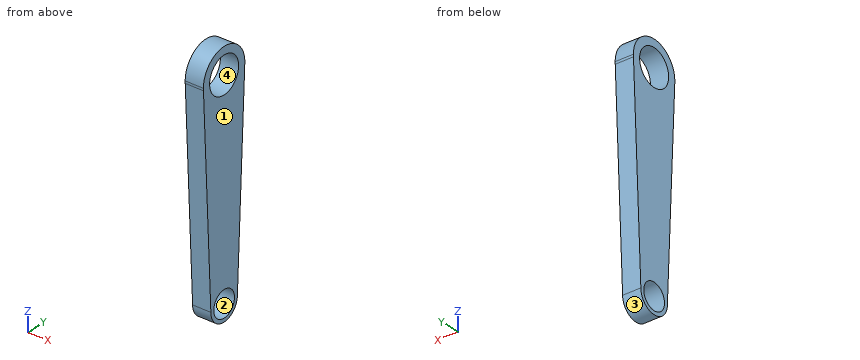
```python
from build123d import *

# Parameters (mm, degrees)
SKETCH_3_R      = 3.5
SKETCH_3_R_2    = 2.5
EXTRUDE_2_DEPTH = 3.5


with BuildPart() as part:
    # 草图3 → 凸台-拉伸2 (new body)
    with BuildSketch(Plane(origin=(0, 0, 0), x_dir=(0, 0, -1), z_dir=(1, 0, 0))):
        with BuildLine():
            Line((0.449090592, 4.979790923), (0, 5))
            ThreePointArc((0, 5), (-5, 0), (0, -5))
            Line((0, -5), (0.449090592, -4.979790923))
            Line((0.449090592, -4.979790923), (40, -3.2))
            ThreePointArc((40, -3.2), (43.2, 0), (40, 3.2))
            Line((40, 3.2), (0.449090592, 4.979790923))
        make_face()
        Circle(SKETCH_3_R, mode=Mode.SUBTRACT)
        with Locations((40, 0)):
            Circle(SKETCH_3_R_2, mode=Mode.SUBTRACT)
    extrude(amount=EXTRUDE_2_DEPTH)


solid = part.part
```
The model under review builds one solid part; all positions refer to its coordinate system, in mm. Face numbers are marked on the shaded views. Round coordinates to 2 decimals unless told otherwise and drop trailing zeros. Order: outer loops, then holes, each group sorted by start corner. A loop starts at its lowest first (then second) coordinate and runs counter-clockwise, first axis right, second up. Notation, with made-up numbers: (-34.5, -39.75) -> (-10.5, -39.75) arc R28 ccw to (-10.5, -7.75) -> close; hole circle Ø4 at (20.25, -27.5). An arc over 180 degrees is marked (long way). Use a Markdown table: item, result.
Q1. For line 1 (Y direction, x = 2.55, z = -40); line 2 (Z direction, x = 1.85, y = 1.25); line 3 (Z direction, x = 2.25, y = 2.25), list the stretches that pass through material, from the lowest coordinate up.
Values:
| item | result |
|---|---|
| line 1 | y = -3.2 to -2.5, 2.5 to 3.2 |
| line 2 | z = -42.95 to -42.17, -37.83 to -3.27, 3.27 to 4.84 |
| line 3 | z = -42.28 to -41.09, -38.91 to -2.68, 2.68 to 4.47 |
Q2. Clearance check with flat-ended pins moving along their axes: P1, Ø5.5, axis at y = 0, z = 0, coming from the -X side; P2, Ø1.5, axis at x = 2, y = 3, coming from the +Z side; P3, Ø1.5, axis at x = 3, z = -15.5, coming from the -Y side; P4, Ø1, axis at y = 0, z = -20.5, coming from the -X side. State where each tip first meets the part, or that it passes through.
Values:
| item | result |
|---|---|
| P1 | passes through |
| P2 | stops at z = 4.47 |
| P3 | stops at y = -4.34 |
| P4 | stops at x = 0 |
Q3. Mouldability with a two-part tool opening along Z and no side actions: class the marked faces 1, 2, 3 and 4 as +Z half, -Z half, draft (parallel to the pull), parting line (faces both ways), or undercut.
Values:
| item | result |
|---|---|
| face 1 | draft |
| face 2 | undercut |
| face 3 | -Z half |
| face 4 | undercut |
Q4. We need section B-B on x = 2.95. Write out the cut boundary in (y, z), then the cut area to 3 significant figures.
Values:
| item | result |
|---|---|
| outline | (-5, 0) -> (-3.2, -40) arc R3.2 ccw to (3.2, -40) -> (5, 0) arc R5 ccw to start; hole circle Ø7 at (0, 0); hole circle Ø5 at (0, -40) |
| area | 325 mm^2 |
Q5. We need section A-A on y = 0. Write out the cut boundary in (x, z), then the cut area to 3 significant figures.
Values:
| item | result |
|---|---|
| outline | (0, -43.2) -> (3.5, -43.2) -> (3.5, -42.5) -> (0, -42.5) -> close; (0, -37.5) -> (3.5, -37.5) -> (3.5, -3.5) -> (0, -3.5) -> close; (0, 3.5) -> (3.5, 3.5) -> (3.5, 5) -> (0, 5) -> close |
| area | 127 mm^2 |
Q6. We need section C-C on z = -20. Write out the cut boundary in (x, y).
Values:
| item | result |
|---|---|
| outline | (0, -4.1) -> (3.5, -4.1) -> (3.5, 4.1) -> (0, 4.1) -> close |
Q7. We need section D-D on y = 2. Write out the cut boundary in (x, z), then the cut area to 3 significant figures.
Values:
| item | result |
|---|---|
| outline | (0, -42.5) -> (3.5, -42.5) -> (3.5, -41.5) -> (0, -41.5) -> close; (0, -38.5) -> (3.5, -38.5) -> (3.5, -2.87) -> (0, -2.87) -> close; (0, 2.87) -> (3.5, 2.87) -> (3.5, 4.58) -> (0, 4.58) -> close |
| area | 134 mm^2 |
